The model under review builds one solid part; all positions refer to its coordinate system, in mm. A direction names the side the tool comes from. Give positions to 0.01 mm unless a question says otherwise; leave off trailing zeros. Write each loop counter-clockwise with the first axis right and the second up, starting at its lowest first coordinate (ties: lowest second). Pieces come first, ordered by that corner, then holes. Notation, with made-up numbers: (32, -6) - (62, -6) arc R28 ccw to (62, 16) - close; hole circle Ø6 at (-2, -37.5). An arc over 180 degrees is marked (long way). Write item = value, one per line.
```python
from build123d import *

# Parameters (mm, degrees)
F0_W     = 52
F0_H     = 13.5
F1_DEPTH = 3
F2_W     = 37.5
F2_H     = 13.5
F2_W_2   = 3
F3_DEPTH = 3
F4_W     = 20
F4_H     = 10
F5_DEPTH = 3


with BuildPart() as f1:
    # F0 (on Front) → F1 (new body)
    with BuildSketch(Plane.XZ):
        with Locations((26, 6.75)):
            Rectangle(F0_W, F0_H)
    extrude(amount=F1_DEPTH)

    # F2 (on face) → F3 (join)
    with BuildSketch(Plane(origin=(0, 0, 0), x_dir=(0, -1, 0), z_dir=(-1, 0, 0))):
        with Locations((-18.75, 6.75)):
            Rectangle(F2_W, F2_H)
        with Locations((1.5, 6.75)):
            Rectangle(F2_W_2, F2_H)
    extrude(amount=F3_DEPTH)

    # F4 (on face) → F5 (join)
    with BuildSketch(Plane.XZ.offset(3)):
        with Locations((18.5, -5)):
            Rectangle(F4_W, F4_H)
    extrude(amount=-F5_DEPTH)


solid = f1.part
```
1. Take a section at B-B on y = 19.5. Give the boundary of the cut face in (x, z), and give its area (3 significant figures).
Findings below:
outline = (-3, 0) - (0, 0) - (0, 13.5) - (-3, 13.5) - close
area = 40.5 mm²
2. For line 1 (Y direction, x = 20.5, z = -0.25), list the stretches that pass through material, from the lowest coordinate up. Write a range as from..to.
Findings below:
line_1 = -3..0
3. Take a section at A-A on z = 6. Give the boundary of the cut face in (x, y), and give its area (4 significant figures).
Findings below:
outline = (-3, -3) - (52, -3) - (52, 0) - (0, 0) - (0, 37.5) - (-3, 37.5) - close
area = 277.5 mm²
4. Machinability: for faces 1 (the flat face through (8.5, -2, -5)), 2 (the flat face through (-1, 37.5, 7)), 3 (the flat face through (25, -3, 4)), 4 (the flat face through (28.5, -2, -5)), 5 (the flat face through (26, 0, 5)), which of the approach directions +Z, -Z, +X, -X, +Y, -Y give a long, thin tool a straight path to every point of the face, cutting with its end or side? Answer none if there is none.
Findings below:
face_1 = -Z, -X, +Y, -Y
face_2 = +Z, -Z, +X, -X, +Y
face_3 = +Z, -Z, +X, -X, -Y
face_4 = -Z, +X, +Y, -Y
face_5 = +Z, -Z, +X, +Y
5. Take a section at C-C on x = 17.5. Give the boundary of the cut face in (y, z).
Findings below:
outline = (-3, -10) - (0, -10) - (0, 13.5) - (-3, 13.5) - close
6. Insertion check: P1, Ø12, axis at x = 19, y = 8, coming from the -Z side; P2, Ø0.9, axis at y = -1.5, z = -4.5, coming from the +X side; P3, Ø3.5, axis at x = 37.5, y = -1.5, coming from the -Z side; P4, Ø4, axis at x = 24.5, z = -3, coming from the +Y side. Each pin has a flat end and moves straight along its axis. Give the tip position at first contact, or say it passes through.
Findings below:
P1 = through
P2 = 28.5
P3 = 0
P4 = 0
